CAD build for the part. Positions are in the model's coordinates, mm. A direction names the side the tool comes from. Give positions to 0.01 mm unless a question says otherwise; leave off trailing zeros. Order: outer loops, then holes, each group sorted by start corner. A loop starts at its lowest first (then second) coordinate and runs counter-clockwise, first axis right, second up.
from build123d import *

# Parameters (mm, degrees)
SKETCH2_R           = 50
BOSS_EXTRUDE1_DEPTH = 25


with BuildPart() as part:
    # Sketch2 → Boss-Extrude1 (new body)
    with BuildSketch(Plane(origin=(0, 0, 0), x_dir=(1, 0, 0), z_dir=(0, 1, 0))):
        with Locations(Location((0, 0, 0), (0, 0, 270))):
            Circle(SKETCH2_R)
        with BuildLine():
            Line((33, 0), (33, 8))
            Line((33, 8), (29.265964208, 8))
            ThreePointArc((29.265964208, 8), (0, 31.404293899), (-29.265964208, 8))
            Line((-29.265964208, 8), (-33, 8))
            Line((-33, 8), (-33, 0))
            Line((-33, 0), (-33, -8))
            Line((-33, -8), (-28.487879111, -8))
            ThreePointArc((-28.487879111, -8), (0, -28.595706101), (28.487879111, -8))
            Line((28.487879111, -8), (33, -8))
            Line((33, -8), (33, 0))
        make_face(mode=Mode.SUBTRACT)
    extrude(amount=-BOSS_EXTRUDE1_DEPTH)


solid = part.part
1. Saw through at B-B on x = 0. Give the cut face in (y, z).
2. Mould opens along X. For faces 1 (the flat face through (31, -12, 8)), 2 (the flat face through (-22, -25, 22)), 3 (the cylindrical face through (15.02, -12.32, 47.69)), 4 (the flat face through (31, -12, -8)) say: released by +X, released by -X, zero draft, split by the parting line, or undercut.
3. Saw through at D-D on x = 41.5. Give the cut face in (y, z).
4. Pin check, flat tips, straight feed: P1, Ø1, axis at y = -13.5, z = -16, coming from the -X side; P2, Ø5, axis at x = 30, y = -16, coming from the -Z side; P3, Ø10, axis at x = -30.5, y = -11, coming from the +Z side. Stop position of each tip, or through.
5. Wall check: line 1 (Z direction, x = 1, y = -14.25); line 2 (X direction, y = -18, z = -27); line 3 (X direction, y = -8.75, z = -17). Give the ranges that are in metal, low to high.
6. Saw through at A-A on z = 0. Give the cut face in (x, y), plus the area to 3 significant figures.
7. Saw through at C-C on y = -14.25. Give the cut face in (x, z), plus the area to 3 significant figures.
8. 3-axis set-ups, long thin cutter, end or side, ignore diameter. For faces 5 (the flat face through (-22, 0, 22)), 6 (the flat face through (-33, -12, 0)): which of +Z, -Z, +X, -X, +Y, -Y reach the whole face in a straight line?
Reported:
1. outline: (-25, -50) - (0, -50) - (0, -31.4) - (-25, -31.4) - close; (-25, 28.6) - (0, 28.6) - (0, 50) - (-25, 50) - close
2. face 1: undercut
2. face 2: zero draft
2. face 3: split by the parting line
2. face 4: undercut
3. outline: (-25, -27.89) - (0, -27.89) - (0, 27.89) - (-25, 27.89) - close
4. P1: stops at x = -47.54
4. P2: stops at z = -41.76
4. P3: stops at z = 43.01
5. line 1: z = -49.99 to -31.39, 28.58 to 49.99
5. line 2: x = -42.08 to -15.65, 15.65 to 42.08
5. line 3: x = -47.02 to -25.63, 25.63 to 47.02
6. outline: (-50, -25) - (-33, -25) - (-33, 0) - (-50, 0) - close; (33, -25) - (50, -25) - (50, 0) - (33, 0) - close
6. area: 850 mm2
7. outline: circle Ø100 at (0, 0); hole (-33, -8) - (-29.27, -8) arc R30 ccw to (29.27, -8) - (33, -8) - (33, 8) - (28.49, 8) arc R30 ccw to (-28.49, 8) - (-33, 8) - close
7. area: 4,920 mm2
8. face 5: +Z, -Z, +X, -X, +Y
8. face 6: +Y, -Y
